Work out the finished part from the listing and answer in its coordinate system (mm). Face numbers are marked on the shaded views. Coordinates: 2 decimals unless noted, no trailing zeros. Write each loop counter-clockwise with the first axis right and the second up, starting at its lowest first coordinate (ties: lowest second). Pieces come first, ordered by that corner, then holes. Notation, with made-up numbers: M 5,83.5 L 60,83.5 A22 ccw 60,99.5 Z; hole C 14.25,52.25 d4. An arc over 180 degrees is marked long. Answer as CSV lines item,"result". Start each with the question number.
(1) The mould has two halves that part along X. Classify the marked faces 1, 2 and 3: released by +X, released by -X, zero draft, split by the parting line, or undercut.
(2) Find the intervals of material crossed by L1, parallel to Y at x = 43, z = 41.6; L2, parallel to X at y = 1, z = 44.35; L3, parallel to X at y = 29, z = 43.65, in increasing order. Write a range as [from, to].
(3) A cutting plane is placed at A-A on y = 5. Give the vertices of the cut face in (x, z), then the cut area to 3 significant figures.
(4) Flat-ended cylindrical pins translate along their axes: P1, Ø3, axis at x = 25.5, z = 44.5, coming from the +Y side; P2, Ø0.8, axis at x = 17.5, z = 42.5, coming from the -Y side; P3, Ø3, axis at y = 5, z = 45.5, coming from the -X side. Find the tip coordinate at first contact, or state that the pin passes through.
from build123d import *

# Parameters (mm, degrees)
M1_START                                       = 40.4
M1_RACK_WITH_INTEGRAL_48_X_44_MM_SEAT_FL_DEPTH = 6
F_56_55_START                                  = 43.1
F_56_55_MM_STOP_SLOT_DEPTH                     = 3.4
FOUR_START                                     = 40.3
FOUR_M3_SEAT_PILOTS_28_X_28_PITCH_PROF_R       = 1.25
FOUR_M3_SEAT_PILOTS_28_X_28_PITCH_DEPTH        = 6.2
SLIDE_START                                    = 40.3
SLIDE_FASTENER_BORES_PROFILE_R                 = 1.1
SLIDE_FASTENER_BORES_DEPTH                     = 6.2
SLIDE_START_2                                  = 44.2
SLIDE_SCREW_RECESSES_PROFILE_R                 = 2.1
SLIDE_SCREW_RECESSES_DEPTH                     = 2.3
RADAR_START                                    = 40.3
RADAR_MOUNTING_SCREW_TOOL_ACCESS_PROFILE_R     = 3.75
RADAR_MOUNTING_SCREW_TOOL_ACCESS_DEPTH         = 6.2


with BuildPart() as part:
    # M1 rack with integral 48 x 44 mm sea 2 → M1 rack with integral 48 x 44 mm seat fl (new body)
    with BuildSketch(Plane.XY.offset(M1_START)):
        Polygon((-69, 10.26), (-68.713242711, 10.26), (-67.908868493, 8.05), (-67.179615611, 8.05), (-66.375241394, 10.26), (-65.571650057, 10.26), (-64.767275839, 8.05), (-64.038022958, 8.05), (-63.23364874, 10.26), (-62.430057404, 10.26), (-61.625683186, 8.05), (-60.896430304, 8.05), (-60.092056086, 10.26), (-59.28846475, 10.26), (-58.484090532, 8.05), (-57.754837651, 8.05), (-56.950463433, 10.26), (-56.146872096, 10.26), (-55.342497879, 8.05), (-54.613244997, 8.05), (-53.808870779, 10.26), (-53.005279443, 10.26), (-52.200905225, 8.05), (-51.471652343, 8.05), (-50.667278126, 10.26), (-49.863686789, 10.26), (-49.059312572, 8.05), (-48.33005969, 8.05), (-47.525685472, 10.26), (-46.722094136, 10.26), (-45.917719918, 8.05), (-45.188467036, 8.05), (-44.384092819, 10.26), (-43.580501482, 10.26), (-42.776127264, 8.05), (-42.046874383, 8.05), (-41.242500165, 10.26), (-40.438908828, 10.26), (-39.634534611, 8.05), (-38.905281729, 8.05), (-38.100907511, 10.26), (-37.297316175, 10.26), (-36.492941957, 8.05), (-35.763689075, 8.05), (-34.959314858, 10.26), (-34.155723521, 10.26), (-33.351349304, 8.05), (-32.622096422, 8.05), (-31.817722204, 10.26), (-31.014130868, 10.26), (-30.20975665, 8.05), (-29.480503768, 8.05), (-28.676129551, 10.26), (-27.872538214, 10.26), (-27.068163996, 8.05), (-26.338911115, 8.05), (-25.534536897, 10.26), (-24.730945561, 10.26), (-23.926571343, 8.05), (-23.197318461, 8.05), (-22.392944243, 10.26), (-21.589352907, 10.26), (-20.784978689, 8.05), (-20.055725808, 8.05), (-19.25135159, 10.26), (-18.447760253, 10.26), (-17.643386036, 8.05), (-16.914133154, 8.05), (-16.109758936, 10.26), (-15.3061676, 10.26), (-14.501793382, 8.05), (-13.7725405, 8.05), (-12.968166283, 10.26), (-12.164574946, 10.26), (-11.360200728, 8.05), (-10.630947847, 8.05), (-9.826573629, 10.26), (-9.022982293, 10.26), (-8.218608075, 8.05), (-7.489355193, 8.05), (-6.684980975, 10.26), (-5.881389639, 10.26), (-5.077015421, 8.05), (-4.34776254, 8.05), (-3.543388322, 10.26), (-2.739796985, 10.26), (-1.935422768, 8.05), (-1.206169886, 8.05), (-0.401795668, 10.26), (0.401795668, 10.26), (1.206169886, 8.05), (1.935422768, 8.05), (2.739796985, 10.26), (3.543388322, 10.26), (4.34776254, 8.05), (5.077015421, 8.05), (5.881389639, 10.26), (6.684980975, 10.26), (7.489355193, 8.05), (8.218608075, 8.05), (9.022982293, 10.26), (9.826573629, 10.26), (10.630947847, 8.05), (11.360200728, 8.05), (12.164574946, 10.26), (12.968166283, 10.26), (13.7725405, 8.05), (14.501793382, 8.05), (15.3061676, 10.26), (16.109758936, 10.26), (16.914133154, 8.05), (17.643386036, 8.05), (18.447760253, 10.26), (19.25135159, 10.26), (20.055725808, 8.05), (20.784978689, 8.05), (21.589352907, 10.26), (22.5, 10.26), (33, -6), (79, -6), (81, -4), (81, 36), (79, 38), (33, 38), (22.5, 22.5), (-69, 22.5), align=None)
    extrude(amount=M1_RACK_WITH_INTEGRAL_48_X_44_MM_SEAT_FL_DEPTH)

    # 56.55 mm stop slot profile → 56.55 mm stop slot (cut)
    with BuildSketch(Plane.XY.offset(F_56_55_START)):
        with BuildLine():
            Line((-56.348667765, 14.8), (-0.2, 14.8))
            ThreePointArc((-0.2, 14.8), (2, 17), (-0.2, 19.2))
            Line((-0.2, 19.2), (-56.348667765, 19.2))
            ThreePointArc((-56.348667765, 19.2), (-58.548667765, 17), (-56.348667765, 14.8))
        make_face()
    extrude(amount=F_56_55_MM_STOP_SLOT_DEPTH, mode=Mode.SUBTRACT)

    # Four M3 seat pilots - 28 x 28 pitch profile → Four M3 seat pilots - 28 x 28 pitch (cut)
    with BuildSketch(Plane.XY.offset(FOUR_START)):
        with Locations(Location((43, 2, 0), (0, 0, 180))):
            Circle(FOUR_M3_SEAT_PILOTS_28_X_28_PITCH_PROF_R)
        with Locations(Location((43, 30, 0), (0, 0, 180))):
            Circle(FOUR_M3_SEAT_PILOTS_28_X_28_PITCH_PROF_R)
        with Locations(Location((71, 2, 0), (0, 0, 180))):
            Circle(FOUR_M3_SEAT_PILOTS_28_X_28_PITCH_PROF_R)
        with Locations(Location((71, 30, 0), (0, 0, 180))):
            Circle(FOUR_M3_SEAT_PILOTS_28_X_28_PITCH_PROF_R)
    extrude(amount=FOUR_M3_SEAT_PILOTS_28_X_28_PITCH_DEPTH, mode=Mode.SUBTRACT)

    # Slide fastener bores profile → Slide fastener bores (cut)
    with BuildSketch(Plane.XY.offset(SLIDE_START)):
        with Locations(Location((5, 19.8, 0), (0, 0, 180))):
            Circle(SLIDE_FASTENER_BORES_PROFILE_R)
        with Locations(Location((15, 19.8, 0), (0, 0, 180))):
            Circle(SLIDE_FASTENER_BORES_PROFILE_R)
    extrude(amount=SLIDE_FASTENER_BORES_DEPTH, mode=Mode.SUBTRACT)

    # Slide screw recesses profile → Slide screw recesses (cut)
    with BuildSketch(Plane.XY.offset(SLIDE_START_2)):
        with Locations((5, 19.8)):
            Circle(SLIDE_SCREW_RECESSES_PROFILE_R)
        with Locations((15, 19.8)):
            Circle(SLIDE_SCREW_RECESSES_PROFILE_R)
    extrude(amount=SLIDE_SCREW_RECESSES_DEPTH, mode=Mode.SUBTRACT)

    # Radar mounting screw tool access profile → Radar mounting screw tool access (cut)
    with BuildSketch(Plane.XY.offset(RADAR_START)):
        with Locations((35.5, -5.5)):
            Circle(RADAR_MOUNTING_SCREW_TOOL_ACCESS_PROFILE_R)
        with Locations((35.5, 37.5)):
            Circle(RADAR_MOUNTING_SCREW_TOOL_ACCESS_PROFILE_R)
        with Locations((78.5, -5.5)):
            Circle(RADAR_MOUNTING_SCREW_TOOL_ACCESS_PROFILE_R)
        with Locations((78.5, 37.5)):
            Circle(RADAR_MOUNTING_SCREW_TOOL_ACCESS_PROFILE_R)
    extrude(amount=RADAR_MOUNTING_SCREW_TOOL_ACCESS_DEPTH, mode=Mode.SUBTRACT)


solid = part.part
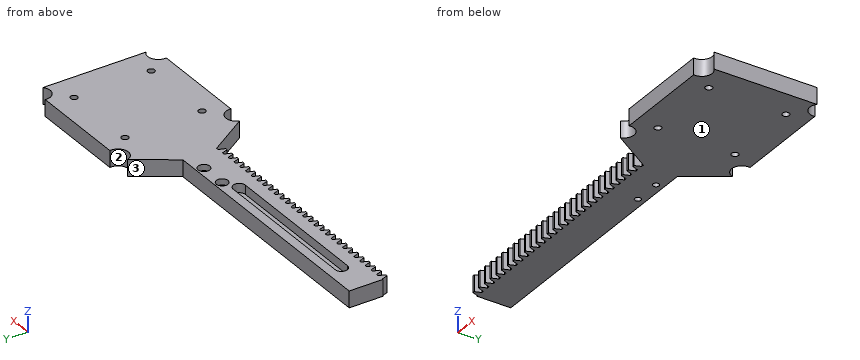
Here are the results:
1,face 1,"zero draft"
1,face 2,"undercut"
1,face 3,"released by -X"
2,L1,"y = [-6, 0.75], [3.25, 28.75], [31.25, 38]"
2,L2,"x = [28.48, 42.25], [43.75, 70.25], [71.75, 81]"
2,L3,"x = [26.9, 42.25], [43.75, 70.25], [71.75, 81]"
3,outline,"M 25.9,40.4 L 81,40.4 L 81,46.4 L 25.9,46.4 Z"
3,area,"331 mm^2"
4,P1,"stops at y = 29.14"
4,P2,"stops at y = 8.05"
4,P3,"stops at x = 24.93"
